Work out the finished part from the listing and answer in its coordinate system (mm). Face numbers are marked on the shaded views. A direction names the side the tool comes from. Give positions to 0.01 mm unless a question says otherwise; leave off trailing zeros. Loops run counter-clockwise (first coordinate to the right, second up) from the corner with the lowest first, then second, coordinate; pieces in that order, holes last. Notation, with made-up numbers: (60.5, 33.25) - (110.5, 33.25) arc R11 cw to (110.5, 44.25) - close; hole circle Ø5 at (-28.75, -30). An arc over 180 degrees is marked (long way). Use CSV: the item, a comma, the result in double quotes.
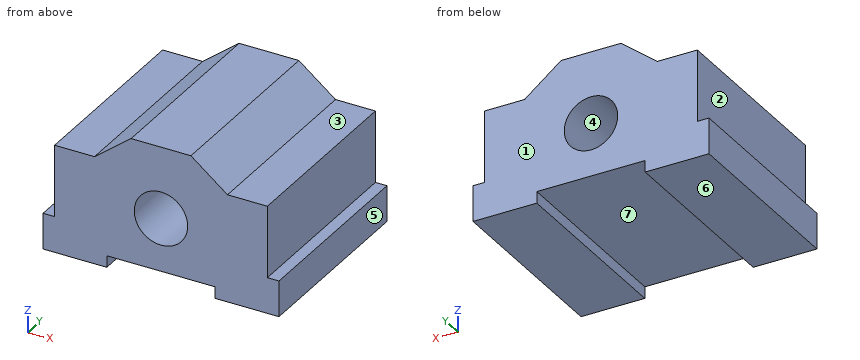
from build123d import *

# Parameters (mm, degrees)
F0_R     = 4.2545
F1_DEPTH = 15.08125


with BuildPart() as f1:
    # F0 (on Front) → F1 (new body, symmetric)
    with BuildSketch(Plane.XZ):
        Polygon((10.588473, 0), (4.7625, 4.572), (0, 4.572), (-4.7625, 4.572), (-10.588473, 0), (-16.938473, 0), (-16.938473, -11.43), (-18.787988, -11.43), (-18.787988, -17.145), (-8.627988, -17.145), (-8.627988, -15.295486), (0, -15.295486), (8.627988, -15.295486), (8.627988, -17.145), (18.787988, -17.145), (18.787988, -11.43), (16.938473, -11.43), (16.938473, 0), align=None)
        with Locations((0, -6.858)):
            Circle(F0_R, mode=Mode.SUBTRACT)
    extrude(amount=F1_DEPTH, both=True)


solid = f1.part
Item 1: Find the intervals of material crossed by line 1 (Z direction, x = 0, y = 4); line 2 (X direction, y = -13.5, z = -7); line 3 (X direction, y = -14, z = -16), in increasing order.
Determined:
line 1,"z = -15.3 to -11.11, -2.6 to 4.57"
line 2,"x = -16.94 to -4.25, 4.25 to 16.94"
line 3,"x = -18.79 to -8.63, 8.63 to 18.79"
Item 2: A cutting plane is placed at D-D on x = -14. Determine the outline of the cut face in (y, z) (3 decimals).
Determined:
outline,"(-15.081, -17.145) - (15.081, -17.145) - (15.081, 0) - (-15.081, 0) - close"
Item 3: A cutting plane is placed at B-B on y = 9. Determine the outline of the cut face in (x, z) (1 decimal).
Determined:
outline,"(-18.8, -17.1) - (-8.6, -17.1) - (-8.6, -15.3) - (8.6, -15.3) - (8.6, -17.1) - (18.8, -17.1) - (18.8, -11.4) - (16.9, -11.4) - (16.9, 0) - (10.6, 0) - (4.8, 4.6) - (-4.8, 4.6) - (-10.6, 0) - (-16.9, 0) - (-16.9, -11.4) - (-18.8, -11.4) - close; hole circle Ø8.5 at (0, -6.9)"
Item 4: For the marked faces 1, 2 and 3, determine the directions among +Z, -Z, +X, -X, +Y, -Y from which every point of the face is accessible in a straight line to the end or side of a thin tool.
Determined:
face 1,"+Z, -Z, +X, -X, +Y"
face 2,"+Z, -X, +Y, -Y"
face 3,"+Z, +X, +Y, -Y"
Item 5: A cutting plane is placed at C-C on z = -5.25. Determine the outline of the cut face in (x, y).
Determined:
outline,"(-16.94, -15.08) - (-3.94, -15.08) - (-3.94, 15.08) - (-16.94, 15.08) - close; (3.94, -15.08) - (16.94, -15.08) - (16.94, 15.08) - (3.94, 15.08) - close"
Item 6: The mould has two halves that part along X. Classify the marked faces 4, 5, 6 and 7: pulls with the +X half, pulls with the -X half, needs draft (parallel to the pull), parting line crosses it, or undercut.
Determined:
face 4,"undercut"
face 5,"pulls with the +X half"
face 6,"needs draft"
face 7,"undercut"
Item 7: A cutting plane is placed at A-A on x = 0. Determine the outline of the cut face in (y, z), and give its area (3 significant figures).
Determined:
outline,"(-15.08, -15.3) - (15.08, -15.3) - (15.08, -11.11) - (-15.08, -11.11) - close; (-15.08, -2.6) - (15.08, -2.6) - (15.08, 4.57) - (-15.08, 4.57) - close"
area,"343 mm²"
Item 8: Given P1, Ø0.6, axis at x = 18, y = 1.5, coming from the +Z side; P2, Ø2, axis at x = -7, y = -4, coming from the -Z side; P3, Ø1.9, axis at x = -13, y = -6.5, coming from the +Z side, each flat-ended and moving along its own axis, determine where each tip first touches the part or whether it passes through.
Determined:
P1,"stops at z = -11.43"
P2,"stops at z = -15.3"
P3,"stops at z = 0"
